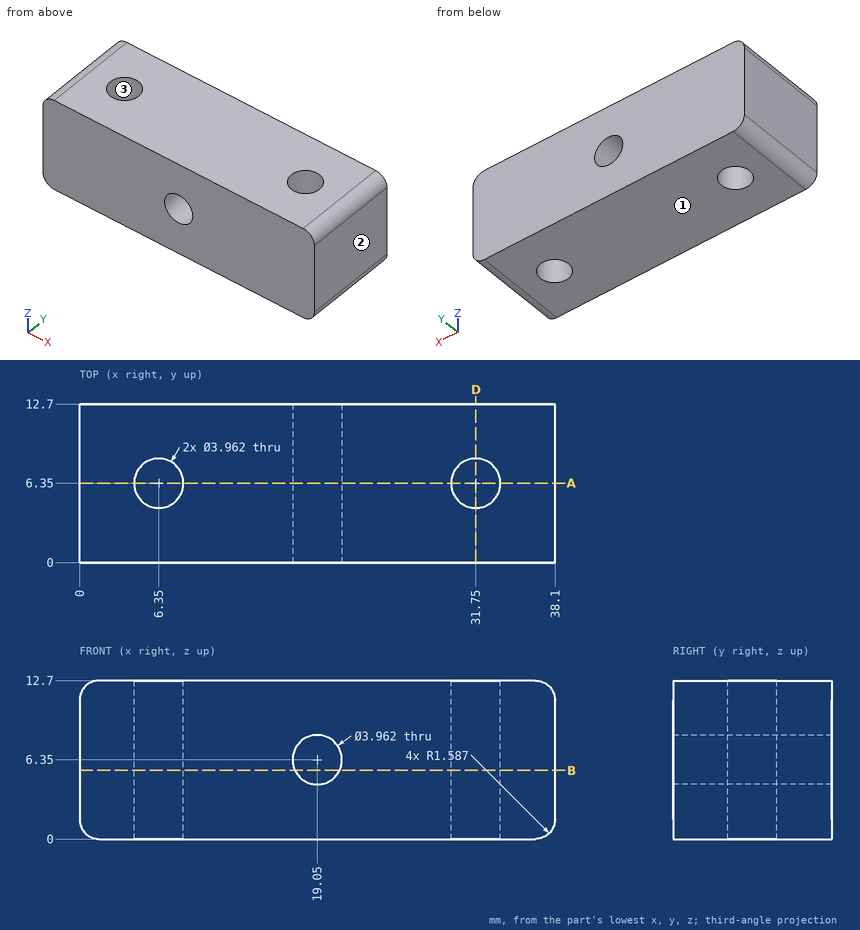
Geometry: see drawing. Coordinates: mm, zero at the bounding-box minimum. Give positions to 0.01 mm unless a question says otherwise; leave off trailing zeros. Loops run counter-clockwise (first coordinate to the right, second up) from the corner with the lowest first, then second, coordinate; pieces in that order, holes last. Notation, with made-up numbers: (-20.5, -27.75) -> (17.5, -27.75) arc R31 ccw to (17.5, 0.25) -> close; hole circle Ø9 at (88, -21.75). An arc over 180 degrees is marked (long way). Put each result on its own line as item: value.
1. Cut plane B-B (z = 5.5). Return the cut outline in (x, y), plus the area to 3 significant figures.
Taken from the geometry:
outline: (0, 0) -> (17.26, 0) -> (17.26, 12.7) -> (0, 12.7) -> close; (20.84, 0) -> (38.1, 0) -> (38.1, 12.7) -> (20.84, 12.7) -> close; hole circle Ø3.96 at (6.35, 6.35); hole circle Ø3.96 at (31.75, 6.35)
area: 414 mm2
2. Pin query (flat end, axial travel): P1, Ø2.5, axis at x = 6.35, y = 6.35, coming from the +Z side. Return the tip coordinate at first contact, or that it passes through.
Taken from the geometry:
P1: passes through
3. Ray query, line 1 along Z through (x, y) = (19, 4.25); line 2 along X through (y, z) = (6.35, 5.25); line 3 along X through (y, z) = (7.5, 7.5) (1 decimal). Return the intervals inside material, ascending. Write a range as [from, to].
Taken from the geometry:
line 1: z = [0, 4.37], [8.33, 12.7]
line 2: x = [0, 4.37], [8.33, 17.4], [20.7, 29.77], [33.73, 38.1]
line 3: x = [0, 4.7], [8, 17.4], [20.7, 30.1], [33.4, 38.1]
4. Pull-direction query (X, two-part tool) for the marked faces 1, 2 and 3; classes: released by +X, released by -X, zero draft, split by the parting line, or undercut.
Taken from the geometry:
face 1: zero draft
face 2: released by +X
face 3: undercut
5. Cut plane D-D (x = 31.75). Return the cut outline in (y, z).
Taken from the geometry:
outline: (0, 0) -> (4.37, 0) -> (4.37, 12.7) -> (0, 12.7) -> close; (8.33, 0) -> (12.7, 0) -> (12.7, 12.7) -> (8.33, 12.7) -> close
6. Cut plane A-A (y = 6.35). Count the separate pieces of the cut face and the enclosed holes in it, plus the area to 3 significant figures.
Taken from the geometry:
separate pieces: 3
enclosed holes: 1
area: 369 mm2
